For this review, take the finished solid that the model builds, in its own axes (mm). A direction names the side the tool comes from. Coordinates: 2 decimals unless noted, no trailing zeros. Write each loop counter-clockwise with the first axis right and the second up, starting at its lowest first coordinate (ties: lowest second). Pieces come first, ordered by that corner, then holes. Notation, with made-up numbers: M -32,38 L -18,38 A21 ccw -18,63 Z; hole C -28.5,-28.75 d5. An arc over 180 degrees is marked long. Return JSON: item names as keys, results as strings.
```python
from build123d import *

# Parameters (mm, degrees)
PAD002_DEPTH = 15
SKETCH005_W  = 87
SKETCH005_H  = 47
SKETCH007_W  = 87
SKETCH007_H  = 47
PAD003_DEPTH = 82


with BuildPart() as part:
    # Sketch004 → Pad002 (new body)
    with BuildSketch(Plane.YZ):
        with BuildLine():
            Line((-25.2, 23.5), (25.2, 23.5))
            ThreePointArc((25.2, -23.5), (27.86, 0), (25.2, 23.5))
            Line((25.2, -23.5), (-25.2, -23.5))
            ThreePointArc((-25.2, 23.5), (-27.86, 0), (-25.2, -23.5))
        make_face()
    extrude(amount=PAD002_DEPTH)

    # Sketch006 (on Face6 of Pad002) → AdditiveLoft001 section 0
    with BuildSketch(Plane.YZ.offset(15)):
        with BuildLine():
            Line((-25.2, 23.5), (25.2, 23.5))
            ThreePointArc((25.2, -23.5), (27.86, 0), (25.2, 23.5))
            Line((-25.2, -23.5), (25.2, -23.5))
            ThreePointArc((-25.2, 23.5), (-27.86, 0), (-25.2, -23.5))
        make_face()
    # Sketch005 → AdditiveLoft001 section 1
    with BuildSketch(Plane.YZ.offset(20)):
        Rectangle(SKETCH005_W, SKETCH005_H)
    loft()

    # Sketch007 (on Face10 of AdditiveLoft001) → Pad003 (join)
    with BuildSketch(Plane.YZ.offset(20)):
        Rectangle(SKETCH007_W, SKETCH007_H)
    extrude(amount=PAD003_DEPTH)


solid = part.part
```
1. We need section A-A (x = 8). State the section outline as (y, z) points.
Checks:
{"outline": "M -25.2,-23.5 L 25.2,-23.5 A105.14 ccw 25.2,23.5 L -25.2,23.5 A105.14 ccw Z"}
2. Wall thickness on L1, parallel to X at y = 34.5, z = -11.5; L2, parallel to X at y = -33, z = 3.5: over which ranges is each line inside the solid? List them lowest first. Write a range as from..to.
Checks:
{"L1": "17.23..102", "L2": "16.66..102"}
3. Clearance check with a flat-ended pin moving along its axis: pin 1 Ø5 at (y, z) = (-28.5, -6.5) entering from -X. State where the tip first meets the part, or that it passes through.
Checks:
{"pin 1": "x = 0"}
4. For faces 1 (the face through (50, -1, -23.5)), 2 (the face through (7.4, 27.86, -0.33)), 3 (the face through (7.4, -27.86, 0.33)), list the 3-axis set-ups (+Z, -Z, +X, -X, +Y, -Y) from which the entire face can be reached by the end or side of a thin tool; tool diameter is ignored.
Checks:
{"face 1": "-Z, +X, -X, +Y, -Y", "face 2": "-X, +Y", "face 3": "-X, -Y"}
